```python
from build123d import *

# Parameters (mm, degrees)
BOSS_EXTRUDE1_DEPTH         = 1.6
SKETCH2_R                   = 3.45
BOSS_EXTRUDE2_DEPTH         = 1.4
TAP_DRILL_FOR_M5X0_8_TAP1_D = 4.2
FILLET2_R                   = 0.3


with BuildPart() as part:
    # Sketch1 → Boss-Extrude1 (new body)
    with BuildSketch(Plane(origin=(0, 0, 0), x_dir=(1, 0, 0), z_dir=(0, 1, 0))):
        with BuildLine():
            Line((1, 0), (14, 0))
            ThreePointArc((14, 0), (14.707106781, 0.292893219), (15, 1))
            Line((15, 1), (15, 9))
            ThreePointArc((15, 9), (14.707106781, 9.707106781), (14, 10))
            Line((14, 10), (1, 10))
            ThreePointArc((1, 10), (0.292893219, 9.707106781), (0, 9))
            Line((0, 9), (0, 1))
            ThreePointArc((0, 1), (0.292893219, 0.292893219), (1, 0))
        make_face()
    extrude(amount=BOSS_EXTRUDE1_DEPTH)

    # Sketch2 → Boss-Extrude2 (add)
    with BuildSketch(Plane(origin=(0, 1.6, 0), x_dir=(1, 0, 0), z_dir=(0, 1, 0))):
        with Locations((7.5, 5)):
            Circle(SKETCH2_R)
    extrude(amount=BOSS_EXTRUDE2_DEPTH)

    # Tap Drill for M5x0.8 Tap1 (through all)
    with Locations(Plane(origin=(7.5, 3, -5), x_dir=(0, 0, 1), z_dir=(0, 1, 0))):
        with Locations((0, 0)):
            Hole(TAP_DRILL_FOR_M5X0_8_TAP1_D / 2)

    # Fillet2
    fillet2_edges = [part.edges().sort_by_distance(p)[0] for p in [
        (14.707106781, 1.6, -0.292893219),
        (7.5, 0, 0),
        (0.292893219, 0, -0.292893219),
        (15, 1.6, -5),
        (14.707106781, 1.6, -9.707106781),
        (7.5, 1.6, -10),
        (0.292893219, 1.6, -9.707106781),
        (4.05, 1.6, -5),
        (4.05, 3, -5),
        (0, 1.6, -5),
        (0.292893219, 1.6, -0.292893219),
        (7.5, 1.6, 0),
        (0, 0, -5),
        (0.292893219, 0, -9.707106781),
        (7.5, 0, -10),
        (14.707106781, 0, -9.707106781),
        (15, 0, -5),
        (14.707106781, 0, -0.292893219),
    ]]
    fillet(fillet2_edges, radius=FILLET2_R)


solid = part.part
```
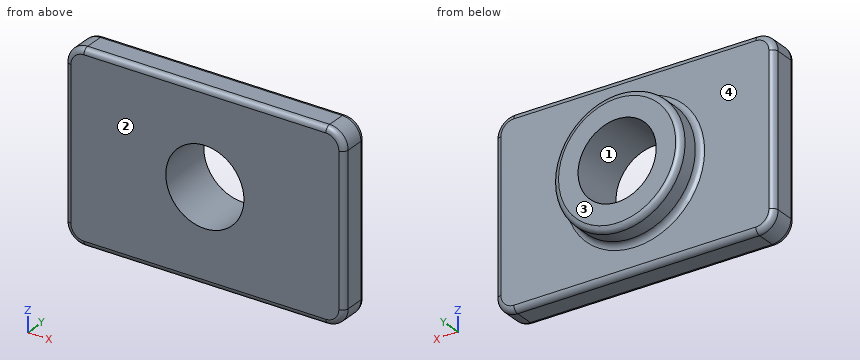
CAD build for the part. Positions are in the model's coordinates, mm. Face numbers are marked on the shaded views. A direction names the side the tool comes from. Round coordinates to 2 decimals unless told otherwise and drop trailing zeros. Loops run counter-clockwise (first coordinate to the right, second up) from the corner with the lowest first, then second, coordinate; pieces in that order, holes last. Notation, with made-up numbers: M 0.5,86.25 L 15.5,86.25 A17 cw 15.5,94.25 Z; hole C 30,77 d9. An arc over 180 degrees is marked long. Return JSON: item names as keys, results as strings. Group by question number.
(1) Saw through at A-A, the plane z = -5. List the corners of the cut face in (x, y), and give its area (3 significant figures).
(2) Saw through at C-C, the plane x = 7.5. List the corners of the cut face in (y, z).
(3) Wall check: probe 1 along X at (y, z) = (1.2, -5); probe 2 along X at (y, z) = (1.95, -5); probe 3 along Y at (x, z) = (9.5, -0.5). Give the ranges that are in metal, low to high. Write a range as [from, to].
(4) Mould opens along X. For the marked faces 1 and 2 say: +X half, -X half, draft (parallel to the pull), parting line (faces both ways), or undercut.
(5) Tool access for the marked faces 3 and 4: list every direction of +Z, -Z, +X, -X, +Y, -Y with a clear straight run to the whole face (end or side of a thin tool).
(6) Saw through at B-B, the plane y = 0.6. List the corners of the cut face in (x, z).
Answer list:
{
 "1": {"outline": "M 0,0.3 A0.3 ccw 0.3,0 L 5.4,0 L 5.4,3 L 4.35,3 A0.3 ccw 4.05,2.7 L 4.05,1.9 A0.3 cw 3.75,1.6 L 0.3,1.6 A0.3 ccw 0,1.3 Z; M 9.6,0 L 14.7,0 A0.3 ccw 15,0.3 L 15,1.3 A0.3 ccw 14.7,1.6 L 11.25,1.6 A0.3 cw 10.95,1.9 L 10.95,2.7 A0.3 ccw 10.65,3 L 9.6,3 Z", "area": "21.0 mm2"},
 "2": {"outline": "M 0,-9.7 A0.3 ccw 0.3,-10 L 1.3,-10 A0.3 ccw 1.6,-9.7 L 1.6,-8.75 A0.3 cw 1.9,-8.45 L 2.7,-8.45 A0.3 ccw 3,-8.15 L 3,-7.1 L 0,-7.1 Z; M 0,-2.9 L 3,-2.9 L 3,-1.85 A0.3 ccw 2.7,-1.55 L 1.9,-1.55 A0.3 cw 1.6,-1.25 L 1.6,-0.3 A0.3 ccw 1.3,0 L 0.3,0 A0.3 ccw 0,-0.3 Z"},
 "3": {"probe 1": "[0, 5.4], [9.6, 15]", "probe 2": "[4.05, 5.4], [9.6, 10.95]", "probe 3": "[0, 1.6]"},
 "4": {"face 1": "undercut", "face 2": "draft"},
 "5": {"face 3": "+Z, -Z, +X, -X, +Y", "face 4": "+Y"},
 "6": {"outline": "M 0,-9 A1 ccw 1,-10 L 14,-10 A1 ccw 15,-9 L 15,-1 A1 ccw 14,0 L 1,0 A1 ccw 0,-1 Z; hole C 7.5,-5 d4.2"}
}
